Design review of the part built by this model. Coordinates are the model's own, in mm. A direction names the side the tool comes from. Round coordinates to 2 decimals unless told otherwise and drop trailing zeros. Loops run counter-clockwise (first coordinate to the right, second up) from the corner with the lowest first, then second, coordinate; pieces in that order, holes last. Notation, with made-up numbers: (9, 30) - (17, 30) arc R20 cw to (17, 61) - close; hole circle Ø7 at (84.25, 61). An arc over 180 degrees is marked (long way). Use one line per item in the form item = value. Start each with the question number.
(1) We need section B-B, the plane y = 1.5. Write out the cut boundary in (x, z) (3 decimals), then the cut area to 3 significant figures.
(2) Wall thickness on probe 1 along X at (y, z) = (-2.75, 2.5) (3 decimals); probe 2 along Z at (x, y) = (-7.5, 0.5); probe 3 along X at (y, z) = (2, -0.5): over which ranges is each line inside the solid? List them lowest first. Write a range as [from, to].
(3) We need section D-D, the plane x = -0.5. Write out the cut boundary in (y, z) (3 decimals), then the cut area to 3 significant figures.
(4) We need section A-A, the plane x = 9. Write out the cut boundary in (y, z) (3 decimals).
(5) The part is to be moulded in two halves that separate along Z. For faces 1 (the flat face through (0, 0, 5.08)), 2 (the flat face through (0, 3.175, 1)), 3 (the flat face through (-9, 0, 2.54)), say which applies: released by +Z, released by -Z, zero draft, split by the parting line, or undercut.
(6) Machinability: for faces 4 (the flat face through (9, 0, 2.54)), 5 (the flat face through (0, 0, -5.08)), which of the approach directions +Z, -Z, +X, -X, +Y, -Y give a long, thin tool a straight path to every point of the face, cutting with its end or side? Answer none if there is none.
(7) We need section C-C, the plane z = 2. Write out the cut boundary in (x, y) (3 decimals).
from build123d import *

# Parameters (mm, degrees)
F0_W     = 21.59
F0_H     = 2.54
F1_DEPTH = 3.175
F2_W     = 11.43
F2_H     = 6.35
F3_DEPTH = 2.54


with BuildPart() as f1:
    # F0 (on Front) → F1 (new body, symmetric)
    with BuildSketch(Plane.XZ):
        Polygon((15.24, -5.08), (15.24, 5.08), (10.725581, 5.08), (10.725581, 2.54), (12.7, 2.54), (12.7, -2.54), (-12.7, -2.54), (-12.7, 2.54), (-10.864419, 2.54), (-10.864419, 5.08), (-15.24, 5.08), (-15.24, -5.08), align=None)
        with Locations((-0.069419, 3.81)):
            Rectangle(F0_W, F0_H)
    extrude(amount=F1_DEPTH, both=True)

    # F2 (on face) → F3 (join)
    with BuildSketch(Plane(origin=(0, 0, 2.54), x_dir=(1, 0, 0), z_dir=(0, 0, -1))):
        Rectangle(F2_W, F2_H)
    extrude(amount=F3_DEPTH)


solid = f1.part
Data:
q1.outline = (-15.24, -5.08) - (15.24, -5.08) - (15.24, 5.08) - (-15.24, 5.08) - close; hole (-12.7, -2.54) - (12.7, -2.54) - (12.7, 2.54) - (5.715, 2.54) - (5.715, 0) - (-5.715, 0) - (-5.715, 2.54) - (-12.7, 2.54) - close
q1.area = 210 mm^2
q2.probe_1 = [-15.24, -12.7], [-5.715, 5.715], [12.7, 15.24]
q2.probe_2 = [-5.08, -2.54], [2.54, 5.08]
q2.probe_3 = [-15.24, -12.7], [12.7, 15.24]
q3.outline = (-3.175, -5.08) - (3.175, -5.08) - (3.175, -2.54) - (-3.175, -2.54) - close; (-3.175, 0) - (3.175, 0) - (3.175, 5.08) - (-3.175, 5.08) - close
q3.area = 48.4 mm^2
q4.outline = (-3.175, -5.08) - (3.175, -5.08) - (3.175, -2.54) - (-3.175, -2.54) - close; (-3.175, 2.54) - (3.175, 2.54) - (3.175, 5.08) - (-3.175, 5.08) - close
q5.face_1 = released by +Z
q5.face_2 = zero draft
q5.face_3 = undercut
q6.face_4 = +Y, -Y
q6.face_5 = -Z, +X, -X, +Y, -Y
q7.outline = (-15.24, -3.175) - (-12.7, -3.175) - (-12.7, 3.175) - (-15.24, 3.175) - close; (-5.715, -3.175) - (5.715, -3.175) - (5.715, 3.175) - (-5.715, 3.175) - close; (12.7, -3.175) - (15.24, -3.175) - (15.24, 3.175) - (12.7, 3.175) - close
